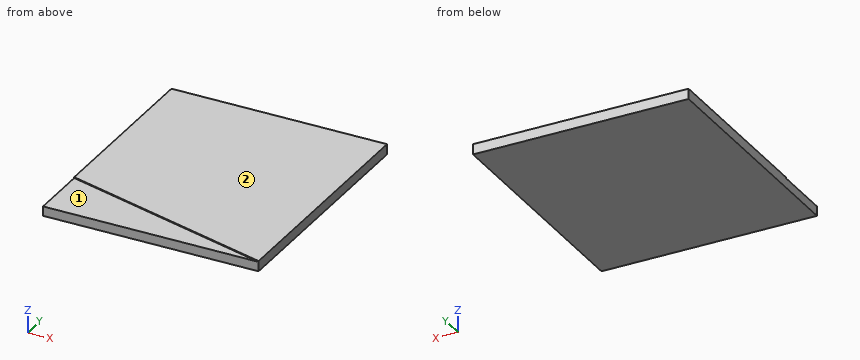
```python
from build123d import *

# Parameters (mm, degrees)
PAD_DEPTH    = 12
POCKET_DEPTH = 1


with BuildPart() as part:
    # Sketch → Pad (new body)
    with BuildSketch(Plane.XY):
        Polygon((0, 0), (0, 140), (250, 140), (250, -140), (0, -140), align=None)
    extrude(amount=PAD_DEPTH)

    # Sketch002 (on Face7 of Pad) → Pocket (cut)
    with BuildSketch(Plane.XY.offset(12)):
        Polygon((0, -140), (0, -71.973152), (250, -140), align=None)
    extrude(amount=-POCKET_DEPTH, mode=Mode.SUBTRACT)


solid = part.part
```
Geometry: final body of the model. Coordinates: model frame, mm. Face numbers are marked on the shaded views. A direction names the side the tool comes from. Round coordinates to 2 decimals unless told otherwise and drop trailing zeros. Order: outer loops, then holes, each group sorted by start corner. A loop starts at its lowest first (then second) coordinate and runs counter-clockwise, first axis right, second up. Notation, with made-up numbers: M 31.5,-3.5 L 61.5,-3.5 A21 ccw 61.5,9.5 Z; hole C 30,6 d1. An arc over 180 degrees is marked long. Use one line per item in the form item = value. Start each with the question number.
Q1. Cut plane A-A (x = 29). Return loops of the section in (y, z), and give its area (3 significant figures).
Q2. Material intervals for line 1 (Y direction, x = 173.5, z = 11.75), sorted ascending. Write a range as [from, to].
Q3. Access query for the marked faces 1 and 2. Directions: +Z, -Z, +X, -X, +Y, -Y. A direction counts if a zero-diameter tool reaches every point of the face in a straight line with its end or side. Return the directions, or none.
Geometry results:
q1.outline = M -140,0 L 140,0 L 140,12 L -79.86,12 L -79.86,11 L -140,11 Z
q1.area = 3,300 mm^2
q2.line_1 = [-119.18, 140]
q3.face_1 = +Z, -X, -Y
q3.face_2 = +Z, +X, -X, +Y, -Y
